Autodesk Inventor part; units mm, degrees
ref_plane "YZ Plane" through (0, 0, 0) normal (1, 0, 0) x (0, 1, 0)
ref_plane "XZ Plane" through (0, 0, 0) normal (0, 1, 0) x (-1, 0, 0)
ref_plane "XY Plane" through (0, 0, 0) normal (0, 0, 1) x (1, 0, 0)
sketch "Grund" plane through (0, 0, 0) normal (0, 1, 0) x (-1, 0, 0)
  line L0 (-43, -43) -> (-7, -43)
  line L1 (-7, -43) -> (-7, -7)
  line L2 (-22.4779, -14.1174) -> (-8.3606, 0)
  line L3 (0, -8.61) -> (-13.9926, -22.6026)
  circle A0 centre (-32.4718, -17.6529) radius 1.5
  line L4 (-18.2353, -22.6026) -> (-22.4779, -18.36)
  line L5 (-22.4779, -14.1174) -> (-22.4779, -18.36)
  line L6 (-13.9926, -22.6026) -> (-18.2353, -22.6026)
  line L7 (-27.5221, -14.1174) -> (-27.5221, -18.36)
  line L8 (-31.7647, -22.6026) -> (-27.5221, -18.36)
  line L9 (-27.5221, -14.1174) -> (-41.6394, 0)
  line L10 (-36.0074, -22.6026) -> (-31.7647, -22.6026)
  line L11 (-50, -8.61) -> (-36.0074, -22.6026)
  line L12 (-27.5221, -35.8826) -> (-27.5221, -31.64)
  line L13 (-27.5221, -35.8826) -> (-41.6394, -50)
  line L14 (-36.0074, -27.3974) -> (-31.7647, -27.3974)
  line L15 (-31.7647, -27.3974) -> (-27.5221, -31.64)
  line L16 (-50, -41.39) -> (-36.0074, -27.3974)
  line L17 (-22.4779, -35.8826) -> (-22.4779, -31.64)
  line L18 (-22.4779, -35.8826) -> (-8.3606, -50)
  line L19 (-18.2353, -27.3974) -> (-22.4779, -31.64)
  line L20 (0, -41.39) -> (-13.9926, -27.3974)
  line L21 (-13.9926, -27.3974) -> (-18.2353, -27.3974)
  circle A1 centre (-32.4718, -32.3471) radius 1.5
  circle A2 centre (-40.25, -40.25) radius 1.5
  line L22 (-43, -7) -> (-43, -43)
  circle A3 centre (-17.5282, -17.6529) radius 1.5
  circle A4 centre (-17.5282, -32.3471) radius 1.5
  circle A5 centre (-9.75, -40.25) radius 1.5
  line L23 (-7, -7) -> (-43, -7)
  circle A6 centre (-9.75, -9.75) radius 1.5
  circle A7 centre (-40.25, -9.75) radius 1.5
  line L24 (0, 0) -> (0, -50)
  line L25 (0, -50) -> (-50, -50)
  line L26 (-50, -50) -> (-50, 0)
  line L27 (-50, 0) -> (0, 0)
  point P0 (-16.114, -25.276)
  point P1 (-24.5992, -33.7613)
  point P2 (-25.4008, -33.7613)
  point P3 (-33.886, -25.276)
  point P4 (-25.4008, -16.2387)
  point P5 (-33.886, -24.724)
  point P6 (-24.5992, -16.2387)
  point P7 (-16.114, -24.724)
  dimension "d0" = 36
  dimension "d1" = 36
  dimension "d4" = 3
  dimension "d5" = 3
  dimension "d6" = 3
  dimension "d7" = 3
  dimension "d9" = 50
  dimension "d10" = 50
extrude "Extrusion1" add sketch "Grund" along normal blind 3
extrude "Extrusion2" add sketch "Grund" along normal blind 7 contours L13 L12 L15 L14 L16 L22 L11 L10 L8 L7 L9 L23 L2 L5 L4 L6 L3 L1 L20 L21 L19 L17 L18 L0 | L0 L18 L25 L13 | L16 L26 L11 L22 | L1 L3 L24 L20 | L9 L27 L2 L23
fillet "Fillet1" radius 2 4 edges at (50, 1.5, -50) (50, 1.5, 0) (0, 1.5, 0) (0, 1.5, -50)
properties part number "Bot 2.1"
Input: part model. Units: mm. Frame: model coordinates. A direction names the side the tool comes from. Coordinates: 2 decimals unless noted, no trailing zeros. Loops run counter-clockwise (first coordinate to the right, second up) from the corner with the lowest first, then second, coordinate; pieces in that order, holes last. Notation, with made-up numbers: (-29, 0.25) - (-23, 0.25) arc R27 cw to (-23, 22.25) - close; hole circle Ø4 at (-30.75, 54). An arc over 180 degrees is marked (long way). Answer in a Markdown table with one row per item. Add a question column.
Item 1: Contact query for a flat-ended pin moving along its axis: P1, Ø5, axis at x = 17.53, z = -17.65, coming from the +Y side. Output: stop coordinate, or through.
Item 2: Mould query, pull axis Z, two halves, no side actions, for faces 1 (the flat face through (50, 3, -25)), 2 (the flat face through (27.522, 5, -16)), 3 (the cylindrical face through (0.6, 1.52, -49.43)). Classes: released by +Z, released by -Z, zero draft, split by the parting line, or undercut.
Item 3: Section query D-D on y = 3.75. Return the cut outline in (x, z), then the cut area to 3 significant figures.
Item 4: Line query: line 1 along Z through (x, y) = (9.75, 2.1); line 2 along X through (y, z) = (6.5, -33.5); line 3 along Z through (x, y) = (33, 5.75). Output: solid intervals per line, ascending. Write a range as [from, to].
Item 5: Section query C-C on x = 9.75. Return the cut outline in (y, z), then the cut area to 3 significant figures.
Item 6: Section query B-B on z = -9.75. Return the cut outline in (x, y), then the cut area to 3 significant figures.
Item 7: Access query for faces 4 (the cylindrical face through (10.075, 1.479, -38.786)), 5 (the flat face through (43.1, 4.97, -34.49)). Directions: +Z, -Z, +X, -X, +Y, -Y. A direction counts if a zero-diameter tool reaches every point of the face in a straight line with its end or side. Return the directions, or none.
Item 8: Section query A-A on x = 44.5. Return the cut outline in (y, z), then the cut area to 3 significant figures.
Recorded:
| question | item | result |
|---|---|---|
| 1 | P1 | y = 3 |
| 2 | face 1 | zero draft |
| 2 | face 2 | undercut |
| 2 | face 3 | released by -Z |
| 3 | outline | (0, -41.39) - (13.99, -27.4) - (18.24, -27.4) - (22.48, -31.64) - (22.48, -35.88) - (8.36, -50) - (41.64, -50) - (27.52, -35.88) - (27.52, -31.64) - (31.76, -27.4) - (36.01, -27.4) - (50, -41.39) - (50, -8.61) - (36.01, -22.6) - (31.76, -22.6) - (27.52, -18.36) - (27.52, -14.12) - (41.64, 0) - (8.36, 0) - (22.48, -14.12) - (22.48, -18.36) - (18.24, -22.6) - (13.99, -22.6) - (0, -8.61) - close |
| 3 | area | 1,290 mm^2 |
| 4 | line 1 | [-50, -41.75], [-38.75, -11.25], [-8.25, 0] |
| 4 | line 2 | [0, 7.89], [22.48, 27.52], [42.11, 50] |
| 4 | line 3 | [-50, -41.36], [-27.4, -22.6], [-8.64, 0] |
| 5 | outline | (0, -50) - (7, -50) - (7, -48.61) - (3, -48.61) - (3, -41.75) - (0, -41.75) - close; (0, -38.75) - (3, -38.75) - (3, -31.64) - (7, -31.64) - (7, -18.36) - (3, -18.36) - (3, -11.25) - (0, -11.25) - close; (0, -8.25) - (3, -8.25) - (3, -1.39) - (7, -1.39) - (7, 0) - (0, 0) - close |
| 5 | area | 196 mm^2 |
| 6 | outline | (0, 0) - (8.25, 0) - (8.25, 3) - (1.14, 3) - (1.14, 7) - (0, 7) - close; (11.25, 0) - (38.75, 0) - (38.75, 3) - (31.89, 3) - (31.89, 7) - (18.11, 7) - (18.11, 3) - (11.25, 3) - close; (41.75, 0) - (50, 0) - (50, 7) - (48.86, 7) - (48.86, 3) - (41.75, 3) - close |
| 6 | area | 196 mm^2 |
| 7 | face 4 | +Y, -Y |
| 7 | face 5 | +Y |
| 8 | outline | (0, -50) - (3, -50) - (3, -35.89) - (7, -35.89) - (7, -14.11) - (3, -14.11) - (3, 0) - (0, 0) - close |
| 8 | area | 237 mm^2 |
